```python
from build123d import *

# Parameters (mm, degrees)
REVOLVE_1_ANGLE     = 180
CUT_EXTRUDE_1_DEPTH = 37.626493144


with BuildPart() as part:
    # Эскиз1 → Повернуть1 (revolve, symmetric)
    with BuildSketch(Plane.XY) as revolve_1_sk:
        Polygon((0, 14.1), (0, 17.5), (2, 17.5), (2, 15), (25, 15), (25, 17.5), (27, 17.5), (27, 14.1), (25.4, 12.5), (1.6, 12.5), align=None)
    revolve(axis=Axis((-27.195971024, 0, 0), (1, 0, 0)), revolution_arc=REVOLVE_1_ANGLE / 2)
    revolve(revolve_1_sk.sketch, axis=Axis((-27.195971024, 0, 0), (-1, 0, 0)), revolution_arc=REVOLVE_1_ANGLE / 2)

    # Эскиз2 → Вырез-Вытянуть1 (cut, through all)
    with BuildSketch(Plane.ZY):
        Polygon((12.85993322, 0), (12.35993322, 1.866025404), (12.35993322, 0), align=None)
        Polygon((-12.85993322, 0), (-12.35993322, 1.866025404), (-12.35993322, 0), align=None)
    extrude(amount=-CUT_EXTRUDE_1_DEPTH, mode=Mode.SUBTRACT)


solid = part.part
```
The model under review builds one solid part; all positions refer to its coordinate system, in mm. A direction names the side the tool comes from. Round coordinates to 2 decimals unless told otherwise and drop trailing zeros. Loops run counter-clockwise (first coordinate to the right, second up) from the corner with the lowest first, then second, coordinate; pieces in that order, holes last.
Item 1: For faces 4 (the face through (13.328, 0.92, 12.613)), 5 (the face through (14, 15, 0)), 6 (the face through (26.014, 17.496, 0.385)), list the 3-axis set-ups (+Z, -Z, +X, -X, +Y, -Y) from which the entire face can be reached by the end or side of a thin tool; tool diameter is ignored.
Determined:
face 4: +X, -X, -Y
face 5: +Y
face 6: +X, -X, +Y
Item 2: Mouldability with a two-part tool opening along Z and no side actions: class faces 1 (the face through (1.014, 17.496, 0.385)), 2 (the face through (27, 15, -1)), 3 (the face through (13.328, 0.92, -12.613)) as released by +Z, released by -Z, zero draft, split by the parting line, or undercut.
Determined:
face 1: split by the parting line
face 2: zero draft
face 3: undercut
Item 3: Take a section at A-A (z = 0). Write out the cut boundary in (x, y).
Determined:
outline: (0, 14.1) - (1.6, 12.5) - (25.4, 12.5) - (27, 14.1) - (27, 17.5) - (25, 17.5) - (25, 15) - (2, 15) - (2, 17.5) - (0, 17.5) - close
Item 4: Take a section at B-B (x = 8.25). Write out the cut boundary in (y, z).
Determined:
outline: (0, -15) arc R15 ccw to (0, 15) - (0, 12.86) - (1.87, 12.36) arc R12.5 cw to (1.87, -12.36) - (0, -12.86) - close
Item 5: For line 1 (X direction, y = 14.5, z = 9); line 2 (Z direction, x = 8, y = 5.25); line 3 (Z direction, x = 17.5, y = 11.25), list the stretches that pass through material, from the lowest coordinate up.
Determined:
line 1: x = 0 to 2, 25 to 27
line 2: z = -14.05 to -11.34, 11.34 to 14.05
line 3: z = -9.92 to -5.45, 5.45 to 9.92
Item 6: Clearance check with flat-ended pins moving along their axes: pin 1 Ø8 at (x, z) = (12, -9.5) entering from +Y; pin 2 Ø4 at (x, y) = (12.5, 13.5) entering from +Z; pin 3 Ø2 at (y, z) = (14.5, -8) entering from -X; pin 4 Ø3 at (x, z) = (18, 9) entering from -Y. State where each tip first meets the part, or that it passes through.
Determined:
pin 1: stops at y = 13.96
pin 2: stops at z = 9.63
pin 3: stops at x = 0
pin 4: stops at y = 6.78
